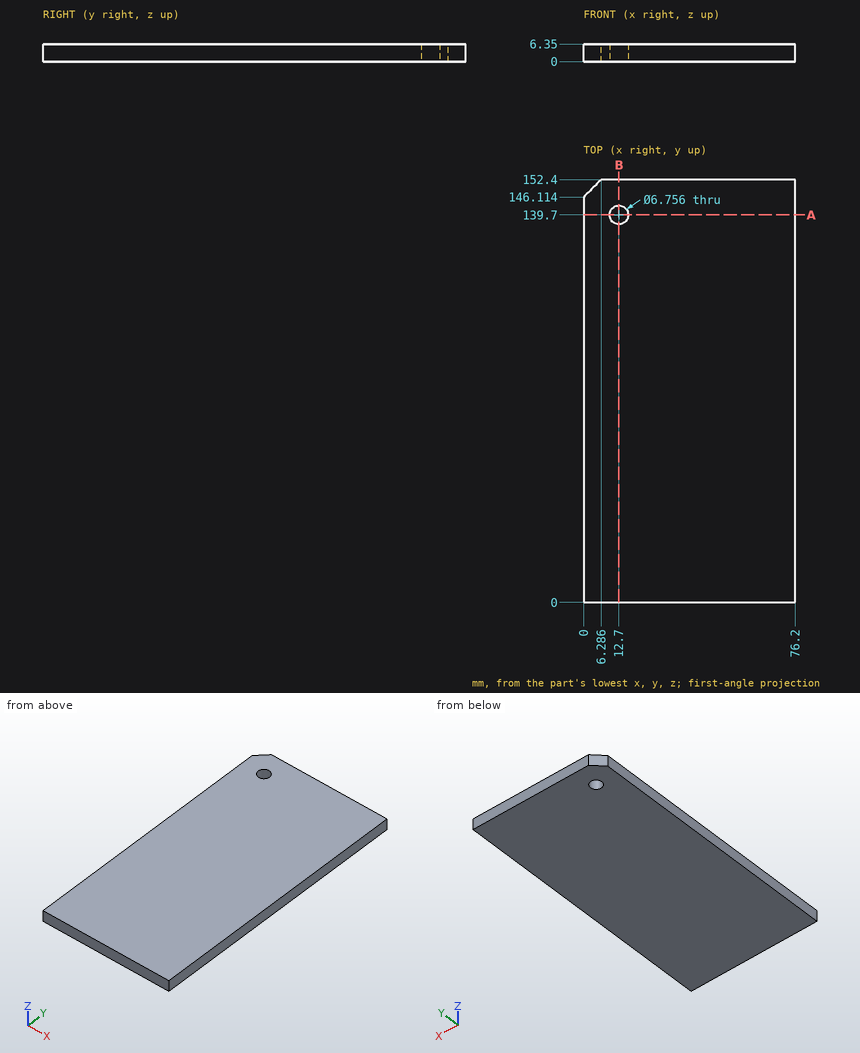
Here's the drawing with two shaded views (mm, measured from the low corner). I have some questions. Coordinates: 2 decimals unless noted, no trailing zeros. Write each loop counter-clockwise with the first axis right and the second up, starting at its lowest first coordinate (ties: lowest second). Pieces come first, ordered by that corner, then holes.
Item 1: Will this pin go through, and if not, where does the flat tip stop? pin 1 (1.5 mm diameter, centred on x = 42.5, y = 82, fed in from -Z).
Item 2: I want a section at B-B on x = 12.7. Write out the boundary of the cut face in (y, z), and give its area (3 significant figures).
Item 3: I want a section at A-A on y = 139.7. Write out the boundary of the cut face in (x, z).
Item 4: If I drill on line 1 (X direction, y = 139.7, z = 4); line 2 (Y direction, x = 12.7, z = 3), over which ranges is the centre line in solid material (lowest first)?
Findings below:
1. pin 1: stops at z = 0
2. outline: (0, 0) - (136.32, 0) - (136.32, 6.35) - (0, 6.35) - close; (143.08, 0) - (152.4, 0) - (152.4, 6.35) - (143.08, 6.35) - close
2. area: 925 mm2
3. outline: (0, 0) - (9.32, 0) - (9.32, 6.35) - (0, 6.35) - close; (16.08, 0) - (76.2, 0) - (76.2, 6.35) - (16.08, 6.35) - close
4. line 1: x = 0 to 9.32, 16.08 to 76.2
4. line 2: y = 0 to 136.32, 143.08 to 152.4
